Geometry: final body of the model. Coordinates: model frame, mm. A direction names the side the tool comes from. Round coordinates to 2 decimals unless told otherwise and drop trailing zeros. Write each loop counter-clockwise with the first axis right and the second up, starting at its lowest first coordinate (ties: lowest second). Pieces come first, ordered by that corner, then holes.
from build123d import *

# Parameters (mm, degrees)
MODEL_R                 = 8.05
MODEL_W                 = 32
MODEL_H                 = 32
SALIENTE_EXTRUIR1_DEPTH = 3
CROQUIS2_W              = 20
CROQUIS2_H              = 3.368375984
SALIENTE_EXTRUIR2_DEPTH = 8
CROQUIS3_R              = 1.5
CORTAR_EXTRUIR1_DEPTH   = 4
REDONDEO1_R             = 2
CROQUIS4_R              = 2.25
CORTAR_EXTRUIR2_DEPTH   = 1


with BuildPart() as part:
    # Model → Saliente-Extruir1 (new body)
    with BuildSketch(Plane.XY):
        with BuildLine():
            Line((89.198959582, -53.020997464), (70.698959583, -53.020997464))
            ThreePointArc((70.698959583, -53.020997464), (69.28474602, -53.606783901), (68.698959582, -55.020997464))
            Line((68.698959582, -55.020997464), (68.698959582, -56.020997464))
            Line((68.698959582, -56.020997464), (48.698959582, -56.020997464))
            Line((48.698959582, -56.020997464), (48.698959583, -55.020997464))
            ThreePointArc((48.698959583, -55.020997464), (48.113173145, -53.606783901), (46.698959582, -53.020997464))
            Line((46.698959582, -53.020997464), (28.198959582, -53.020997464))
            ThreePointArc((28.198959582, -53.020997464), (26.78474602, -52.435211026), (26.198959582, -51.020997464))
            Line((26.198959582, -51.020997464), (26.198959582, 28.005161342))
            ThreePointArc((26.198959582, 28.005161342), (28.72866076, 33.955350752), (34.23516159, 37.343947904))
            ThreePointArc((34.23516159, 37.343947904), (33.593436695, 34.698271666), (34.088137303, 32.021205191))
            ThreePointArc((34.088137303, 32.021205191), (39.416934224, 36.659890309), (46.05573433, 39.07646007))
            ThreePointArc((46.05573433, 39.07646007), (45.031738366, 36.571712032), (46.078788199, 34.076513218))
            ThreePointArc((46.078788199, 34.076513218), (50.656295588, 37.451644327), (56.004342405, 39.386451589))
            ThreePointArc((56.004342405, 39.386451589), (58.081757107, 34.687776201), (62.041164818, 31.41420127))
            ThreePointArc((62.041164818, 31.41420127), (70.12810034, 36.137425043), (79.321724733, 37.92198087))
            ThreePointArc((79.321724733, 37.92198087), (82.046795326, 30.144055291), (89.601066614, 26.849344169))
            ThreePointArc((89.601066614, 26.849344169), (90.596172101, 26.096573111), (91.198959583, 25.004077597))
            Line((91.198959583, 25.004077597), (91.198959583, -51.020997464))
            ThreePointArc((91.198959583, -51.020997464), (90.613173145, -52.435211026), (89.198959582, -53.020997464))
        make_face()
        with Locations((71.698959582, 14.979002536)):
            Circle(MODEL_R, mode=Mode.SUBTRACT)
        with Locations((45.698959583, 14.979002536)):
            Circle(MODEL_R, mode=Mode.SUBTRACT)
        with Locations((58.698959582, -17.020997464)):
            Rectangle(MODEL_W, MODEL_H, mode=Mode.SUBTRACT)
    extrude(amount=-SALIENTE_EXTRUIR1_DEPTH)

    # Croquis2 → Saliente-Extruir2 (add)
    with BuildSketch(Plane(origin=(0, 0, -3), x_dir=(-1, 0, 0), z_dir=(0, 0, -1))):
        with Locations((-58.698959582, -54.336809472)):
            Rectangle(CROQUIS2_W, CROQUIS2_H)
    extrude(amount=SALIENTE_EXTRUIR2_DEPTH)

    # Croquis3 → Cortar-Extruir1 (cut)
    with BuildSketch(Plane(origin=(0, -52.65262148, 0), x_dir=(1, 0, 0), z_dir=(0, 1, 0))):
        with Locations((64.698959582, 6.5)):
            Circle(CROQUIS3_R)
        with Locations((52.698959582, 6.5)):
            Circle(CROQUIS3_R)
    extrude(amount=-CORTAR_EXTRUIR1_DEPTH, mode=Mode.SUBTRACT)

    # Redondeo1
    redondeo1_edges = [part.edges().sort_by_distance(p)[0] for p in [
        (48.698959582, -54.336809472, -11),
        (68.698959582, -54.336809472, -11),
    ]]
    fillet(redondeo1_edges, radius=REDONDEO1_R)

    # Croquis4 → Cortar-Extruir2 (cut)
    with BuildSketch(Plane(origin=(0, -52.65262148, 0), x_dir=(1, 0, 0), z_dir=(0, 1, 0))):
        with Locations((52.698959582, 6.5)):
            Circle(CROQUIS4_R)
        with Locations((64.698959582, 6.5)):
            Circle(CROQUIS4_R)
    extrude(amount=-CORTAR_EXTRUIR2_DEPTH, mode=Mode.SUBTRACT)


solid = part.part
1) Reachability of faces 4 (the flat face through (59, -52.653, -7)), 5 (the flat face through (80, -53.021, -1)), 6 (the flat face through (68.699, -54, -5)), 7 (the cylindrical face through (45.03, 36.61, -1.48)), 8 (the cylindrical face through (62.45, -53.15, -6.6)) from +Z, -Z, +X, -X, +Y, -Y: full face, straight path, thin tool, end or side. Return the list, or none.
2) Section B-B on z = -6.5. Output: boundary loops of the cut face in (x, y), plus the area to 3 significant figures.
3) Section D-D on y = 20.5. Output: boundary loops of the cut face in (x, z), plus the area to 3 significant figures.
4) Section C-C on x = 39.5. Output: boundary loops of the cut face in (y, z).
5) Line query: probe 1 along X at (y, z) = (-55.25, -6.5); probe 2 along X at (y, z) = (-52.9, -6.5); probe 3 along Y at (x, z) = (59, -10). Output: solid intervals per line, ascending.
6) Section A-A on y = -2.5. Output: boundary loops of the cut face in (x, z), plus the area to 3 significant figures.
7) First-contact query: P1, Ø4, axis at x = 52.7, z = -6.5, coming from the +Y side; P2, Ø2.5, axis at y = -55, z = -5, coming from the -X side; P3, Ø3, axis at x = 72.5, z = -3, coming from the +Y side. Flat tips, straight axial feed; report the tip coordinate or a pass-through.
8) Draft query along Y for faces 1 (the cylindrical face through (28.669, 33.885, -1.479)), 2 (the cylindrical face through (68.13, -54.31, -10.4)), 3 (the cylindrical face through (79.135, 11.896, -1.479)). Return one class per face: pulls with the +Y half, pulls with the -Y half, needs draft (parallel to the pull), parting line crosses it, or undercut.
Filled in:
1. face 4: -Z, +X, -X, +Y
1. face 5: +Z, -Z, +X, -Y
1. face 6: -Z, +X, -Y
1. face 7: +Z, -Z
1. face 8: +Y
2. outline: (48.7, -56.02) - (51.2, -56.02) - (51.2, -53.65) - (50.45, -53.65) - (50.45, -52.65) - (48.7, -52.65) - close; (54.2, -56.02) - (63.2, -56.02) - (63.2, -53.65) - (62.45, -53.65) - (62.45, -52.65) - (54.95, -52.65) - (54.95, -53.65) - (54.2, -53.65) - close; (66.2, -56.02) - (68.7, -56.02) - (68.7, -52.65) - (66.95, -52.65) - (66.95, -53.65) - (66.2, -53.65) - close
2. area: 44.2 mm2
3. outline: (26.2, -3) - (39.84, -3) - (39.84, 0) - (26.2, 0) - close; (51.56, -3) - (65.84, -3) - (65.84, 0) - (51.56, 0) - close; (77.56, -3) - (91.2, -3) - (91.2, 0) - (77.56, 0) - close
3. area: 125 mm2
4. outline: (-53.02, -3) - (9.84, -3) - (9.84, 0) - (-53.02, 0) - close; (20.11, -3) - (36.71, -3) - (36.71, 0) - (20.11, 0) - close
5. probe 1: x = 48.7 to 51.2, 54.2 to 63.2, 66.2 to 68.7
5. probe 2: x = 48.7 to 50.45, 54.95 to 62.45, 66.95 to 68.7
5. probe 3: y = -56.02 to -52.65
6. outline: (26.2, -3) - (42.7, -3) - (42.7, 0) - (26.2, 0) - close; (74.7, -3) - (91.2, -3) - (91.2, 0) - (74.7, 0) - close
6. area: 99.0 mm2
7. P1: stops at y = -53.65
7. P2: stops at x = 48.7
7. P3: stops at y = 37.28
8. face 1: pulls with the +Y half
8. face 2: needs draft
8. face 3: undercut
